```python
from build123d import *

# Parameters (mm, degrees)
SKETCH1_R           = 24
BOSS_EXTRUDE1_DEPTH = 8
SKETCH2_R           = 17.6
CUT_EXTRUDE1_DEPTH  = 16
CUT_EXTRUDE2_START  = -5.1
SKETCH3_W           = 10.2
SKETCH3_H           = 96
CUT_EXTRUDE2_DEPTH  = 15.1
SKETCH4_R           = 1.6
CUT_EXTRUDE3_DEPTH  = 60


with BuildPart() as part:
    # Sketch1 → Boss-Extrude1 (new, symmetric)
    with BuildSketch(Plane(origin=(0, 0, 0), x_dir=(1, 0, 0), z_dir=(0, 1, 0))):
        with Locations(Location((0, 0, 0), (0, 0, 270))):
            Circle(SKETCH1_R)
    extrude(amount=BOSS_EXTRUDE1_DEPTH, both=True)

    # Sketch2 → Cut-Extrude1 (cut, symmetric)
    with BuildSketch(Plane(origin=(0, 0, 0), x_dir=(1, 0, 0), z_dir=(0, 1, 0))):
        with Locations(Location((0, 0, 0), (0, 0, 270))):
            Circle(SKETCH2_R)
    extrude(amount=CUT_EXTRUDE1_DEPTH, both=True, mode=Mode.SUBTRACT)

    # Sketch3 → Cut-Extrude2 (cut)
    with BuildSketch(Plane(origin=(0, 0, 0), x_dir=(1, 0, 0), z_dir=(0, 1, 0)).offset(CUT_EXTRUDE2_START)):
        with Locations((21.9, 0)):
            Rectangle(SKETCH3_W, SKETCH3_H)
    extrude(amount=CUT_EXTRUDE2_DEPTH, mode=Mode.SUBTRACT)

    # Sketch4 → Cut-Extrude3 (cut, symmetric)
    with BuildSketch(Plane(origin=(0, 0, 0), x_dir=(0, 0, -1), z_dir=(1, 0, 0))):
        Circle(SKETCH4_R)
    extrude(amount=CUT_EXTRUDE3_DEPTH, both=True, mode=Mode.SUBTRACT)


solid = part.part
```
The listing builds one solid part. Answer for the finished solid, in the listing's coordinates (mm). A direction names the side the tool comes from. Round coordinates to 2 decimals unless told otherwise and drop trailing zeros. Order: outer loops, then holes, each group sorted by start corner. A loop starts at its lowest first (then second) coordinate and runs counter-clockwise, first axis right, second up. Notation, with made-up numbers: (55, 65) - (110, 65) arc R13 cw to (110, 83) - close; hole circle Ø7 at (28.5, 65). An arc over 180 degrees is marked (long way). Put each result on its own line as item: value. Start each with the question number.
(1) For faces 5 (the flat face through (13, -8, -13)), 6 (the flat face through (16.8, 1, 11)), determine the directions among +Z, -Z, +X, -X, +Y, -Y from which every point of the face is accessible in a straight line to the end or side of a thin tool.
(2) Find section B-B (z = 0). Give the vertices of the cut face in (x, y), plus the area to 3 significant figures.
(3) Find section C-C (z = -12.5). Give the vertices of the cut face in (x, y), plus the area to 3 significant figures.
(4) Determine the mould class of faces 1 (the cylindrical face through (-15.614, 0.112, 8.121)), 2 (the flat face through (16.8, 1, -11)), 3 (the flat face through (-19, 8, 0)), 4 (the cylindrical face through (-23.43, 0.11, -5.2)) for opening direction X: released by +X, released by -X, zero draft, split by the parting line, or undercut.
(5) Find section A-A (x = 0). Give the vertices of the cut face in (y, z).
(6) Given P1, Ø4, axis at x = 10, y = -0.5, coming from the +Z side; P2, Ø8, axis at x = 16, y = 1.5, coming from the +Z side; P3, Ø3.5, axis at x = 21.5, z = 5, coming from the +Y side; P4, Ø3, axis at y = 0, z = 0, coming from the -X side, each flat-ended and moving along its own axis, determine where each tip first touches the part or whether it passes through.
(7) Straight lines are drawn through the part: probe 1 along Y at (x, z) = (-22, 0); probe 2 along X at (y, z) = (-7, 0); probe 3 along Z at (x, y) = (-0.5, -2.5). For each, find the intervals that lie inside material, in ascending order. Write a range as from..to.
(8) Find section D-D (y = -6.5). Give the vertices of the cut face in (x, z), plus the area to 3 significant figures.
Reply:
1. face 5: +Z, -Z, +X, -X, -Y
1. face 6: +Z, -Z, +X, +Y
2. outline: (-24, -8) - (-17.6, -8) - (-17.6, -1.6) - (-24, -1.6) - close; (-24, 1.6) - (-17.6, 1.6) - (-17.6, 8) - (-24, 8) - close; (17.6, -8) - (24, -8) - (24, -5.1) - (17.6, -5.1) - close
2. area: 100 mm^2
3. outline: (-20.49, -8) - (-12.39, -8) - (-12.39, 8) - (-20.49, 8) - close; (12.39, -8) - (20.49, -8) - (20.49, -5.1) - (16.8, -5.1) - (16.8, 8) - (12.39, 8) - close
3. area: 211 mm^2
4. face 1: undercut
4. face 2: released by +X
4. face 3: zero draft
4. face 4: split by the parting line
5. outline: (-8, -24) - (8, -24) - (8, -17.6) - (-8, -17.6) - close; (-8, 17.6) - (8, 17.6) - (8, 24) - (-8, 24) - close
6. P1: z = 22.63
6. P2: z = 20.78
6. P3: y = -5.1
6. P4: through
7. probe 1: -8..-1.6, 1.6..8
7. probe 2: -24..-17.6, 17.6..24
7. probe 3: -23.99..-17.59, 17.59..23.99
8. outline: circle Ø48 at (0, 0); hole circle Ø35.2 at (0, 0)
8. area: 836 mm^2
